from build123d import *

# Parameters (mm, degrees)
SKETCH1_W           = 101.6
SKETCH1_H           = 69.85
BOSS_EXTRUDE1_DEPTH = 3.302
SKETCH4_R           = 1.5875
CUT_EXTRUDE1_DEPTH  = 4.302
FILLET1_R           = 5
SKETCH5_R           = 4.064
CUT_EXTRUDE2_DEPTH  = 4.302


with BuildPart() as part:
    # Sketch1 → Boss-Extrude1 (new body)
    with BuildSketch(Plane(origin=(0, 0, 0), x_dir=(1, 0, 0), z_dir=(0, 1, 0))):
        Rectangle(SKETCH1_W, SKETCH1_H)
    extrude(amount=BOSS_EXTRUDE1_DEPTH)

    # Sketch4 → Cut-Extrude1 (cut, through all)
    with BuildSketch(Plane(origin=(0, 0, 0), x_dir=(-1, 0, 0), z_dir=(0, -1, 0))):
        with Locations((0, 31.75)):
            Circle(SKETCH4_R)
        with Locations((-47.625, 0)):
            Circle(SKETCH4_R)
        with Locations((0, -31.75)):
            Circle(SKETCH4_R)
        with Locations((47.625, 0)):
            Circle(SKETCH4_R)
    extrude(amount=-CUT_EXTRUDE1_DEPTH, mode=Mode.SUBTRACT)

    # Fillet1
    fillet1_edges = [part.edges().sort_by_distance(p)[0] for p in [
        (50.8, 1.651, 34.925),
        (-50.8, 1.651, 34.925),
        (-50.8, 1.651, -34.925),
        (50.8, 1.651, -34.925),
    ]]
    fillet(fillet1_edges, radius=FILLET1_R)

    # Sketch5 → Cut-Extrude2 (cut, through all)
    with BuildSketch(Plane(origin=(0, 3.302, 0), x_dir=(1, 0, 0), z_dir=(0, 1, 0))):
        with Locations((-6.671406789, -4.328326436)):
            Circle(SKETCH5_R)
    extrude(amount=-CUT_EXTRUDE2_DEPTH, mode=Mode.SUBTRACT)


solid = part.part
Check sheet for the modelled part. Datum: model origin and axes. Units: mm. Round coordinates to 2 decimals unless told otherwise and drop trailing zeros. Loops run counter-clockwise (first coordinate to the right, second up) from the corner with the lowest first, then second, coordinate; pieces in that order, holes last.
1. Sectioned sample at B-B on z = -31.75. Record the boundary of the cut face in (x, y).
2. Sectioned sample at A-A on x = 0. Record the boundary of the cut face in (y, z) (1 decimal), and give its area (3 significant figures).
3. Scan lines: probe 1 along Z at (x, y) = (-5, 1.3) (3 decimals); probe 2 along X at (y, z) = (2.8, -30.5); probe 3 along Z at (x, y) = (-3, 0.65) (3 decimals). Record each from-to range of solid material in increasing order.
4. Mould release check, pull along Z, two halves, no side actions. Record for faces 1 (the cylindrical face through (-0.85, 1.63, 30.41)), 2 (the flat face through (-50.8, 2, 0)), 3 (the cylindrical face through (49.296, 1.674, -33.499)): released by +Z, released by -Z, zero draft, split by the parting line, or undercut.
Recorded:
1. outline: (-50.46, 0) - (-1.59, 0) - (-1.59, 3.3) - (-50.46, 3.3) - close; (1.59, 0) - (50.46, 0) - (50.46, 3.3) - (1.59, 3.3) - close
2. outline: (0, -34.9) - (3.3, -34.9) - (3.3, -33.3) - (0, -33.3) - close; (0, -30.2) - (3.3, -30.2) - (3.3, 30.2) - (0, 30.2) - close; (0, 33.3) - (3.3, 33.3) - (3.3, 34.9) - (0, 34.9) - close
2. area: 210 mm2
3. probe 1: z = -34.925 to 0.624, 8.033 to 34.925
3. probe 2: x = -50.77 to -0.98, 0.98 to 50.77
3. probe 3: z = -34.925 to 2.586, 6.071 to 34.925
4. face 1: undercut
4. face 2: zero draft
4. face 3: released by -Z
